```python
from build123d import *

# Parameters (mm, degrees)
F1_DEPTH      = 15.875
F0_R          = 12.7
F3_END_RADIUS = 12.7
F2_R          = 12.7
F3_REACH      = 874.1220244843
F7_R          = 6.35
F8_DEPTH      = 50.8


# Not quite as in the source:
# - a feature of the source that left no trace in its solid (it failed there, or was rolled back) is left out


with BuildPart() as f1:
    # F0 (on Front) → F1 (new body, symmetric)
    with BuildSketch(Plane.XZ):
        with BuildLine():
            ThreePointArc((838.2, 0), (825.5, 12.7), (812.8, 0))
            ThreePointArc((812.8, 0), (825.5, -12.7), (838.2, 0))
        make_face()
        with BuildLine():
            ThreePointArc((819.15, 0), (825.5, 6.35), (831.85, 0))
            ThreePointArc((831.85, 0), (825.5, -6.35), (819.15, 0))
        make_face(mode=Mode.SUBTRACT)
    extrude(amount=F1_DEPTH, both=True)



with BuildPart() as f1b:
    # F0 (on Front) → F1, piece 2 (new body, symmetric)
    with BuildSketch(Plane.XZ):
        Circle(F0_R)
    extrude(amount=F1_DEPTH, both=True)


with BuildPart() as f1_1:
    add(f1.part)

    add(f1b.part)  # F3 merges F1b
    f3_end = (Plane(origin=(825.5, 7.9375, 0), x_dir=(0, 0, -1), z_dir=(0, -1, 0)) * Cylinder(F3_END_RADIUS, 3451.9858515901, mode=Mode.PRIVATE)).faces().sort_by_distance((825.5, 7.9375, 12.7))[0]
    # F2 (on Right) → F3 (join, up to the whole of a round face its end follows)
    with BuildSketch(Plane.YZ):
        Circle(F2_R)
    f3_long = extrude(amount=F3_REACH, mode=Mode.PRIVATE)
    add(split(f3_long, bisect_by=f3_end, keep=Keep.ALL, mode=Mode.PRIVATE).solids().sort_by_distance((0, 0, 0))[0])

    # F7 (on face) → F8 (cut)
    with BuildSketch(Plane.XZ.offset(15.875)):
        Circle(F7_R)
    extrude(amount=-F8_DEPTH, mode=Mode.SUBTRACT)


solid = f1_1.part
```
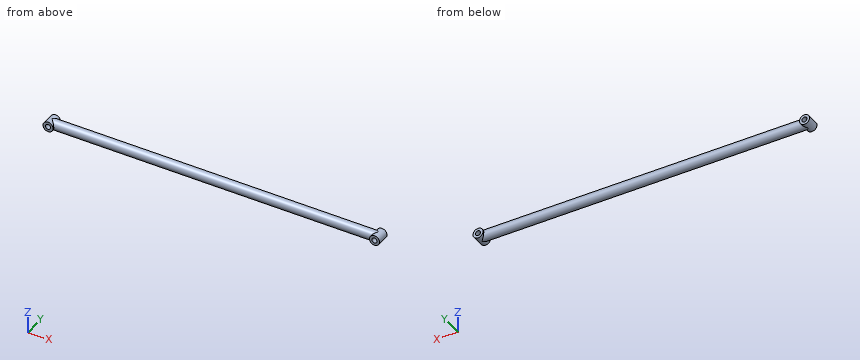
CAD build for the part. Positions are in the model's coordinates, mm. Give positions to 0.01 mm unless a question says otherwise; leave off trailing zeros. Loops run counter-clockwise (first coordinate to the right, second up) from the corner with the lowest first, then second, coordinate; pieces in that order, holes last. Notation, with made-up numbers: M 3.25,4 L 45.25,4 A16 ccw 45.25,34 Z; hole C 35.5,39 d9. An arc over 180 degrees is marked long. Use one line per item in the form item = value.
Item 1: Slice it at C-C (x = 717). List the corners of the cut face in (y, z).
Determined:
outline = C 0,0 d25.4
Item 2: Drill centre lines: probe 1 along X at (y, z) = (5, 0.5); probe 2 along Z at (x, y) = (0, 2); probe 3 along X at (y, z) = (1.5, 4.25). Where is each one in solid material? Low to high. Write a range as from..to.
Determined:
probe_1 = -12.69..-6.33, 6.33..819.17, 831.83..838.19
probe_2 = -12.7..-6.35, 6.35..12.7
probe_3 = -11.97..-4.72, 4.72..820.78, 830.22..837.47
Item 3: Flat gauge pins, fed straight in: pin 1 (1 mm diameter, centred on x = 507.5, y = -2.5, fed in from -Z); pin 2 (10 mm diameter, centred on x = 825.5, z = 0, fed in from +Y); pin 3 (3 mm diameter, centred on x = 181.5, y = -9.5, fed in from +Z); pin 4 (2 mm diameter, centred on x = 567.5, y = 9.5, fed in from -Z). Where does each tip first touch, or does it go through?
Determined:
pin_1 = -12.54
pin_2 = through
pin_3 = 9.86
pin_4 = -9.44
Item 4: Slice it at A-A (z = 0). List the corners of the cut face in (x, y) (3 decimals).
Determined:
outline = M -12.7,-15.875 L -6.35,-15.875 L -6.35,15.875 L -12.7,15.875 Z; M 6.35,-15.875 L 12.7,-15.875 L 12.7,-12.7 L 812.8,-12.7 L 812.8,-15.875 L 819.15,-15.875 L 819.15,15.875 L 812.8,15.875 L 812.8,12.7 L 12.7,12.7 L 12.7,15.875 L 6.35,15.875 Z; M 831.85,-15.875 L 838.2,-15.875 L 838.2,15.875 L 831.85,15.875 Z
Item 5: Slice it at B-B (y = 0). List the corners of the cut face in (x, z).
Determined:
outline = M 0,-12.7 L 825.5,-12.7 A12.7 ccw 825.5,12.7 L 0,12.7 A12.7 ccw Z; hole C 0,0 d12.7; hole C 825.5,0 d12.7
